```python
from build123d import *

# Parameters (mm, degrees)
SKETCH1_W           = 64
SKETCH1_H           = 54.105
BOSS_EXTRUDE1_DEPTH = 12
SKETCH2_R           = 3.15
CUT_EXTRUDE1_DEPTH  = 85.660209219
FILLET1_R           = 8
SKETCH3_R           = 11
SKETCH3_R_2         = 1.7
CUT_EXTRUDE2_DEPTH  = 85.660209219
CUT_EXTRUDE4_DEPTH  = 8
CUT_EXTRUDE5_START  = -85.903698808
SKETCH6_R           = 3.05
CUT_EXTRUDE5_DEPTH  = 93.903698808


with BuildPart() as part:
    # Sketch1 → Boss-Extrude1 (new body)
    with BuildSketch(Plane.XY):
        with Locations((32, 27.0525)):
            Rectangle(SKETCH1_W, SKETCH1_H)
    extrude(amount=BOSS_EXTRUDE1_DEPTH)

    # Sketch2 → Cut-Extrude1 (cut, through all)
    with BuildSketch(Plane(origin=(0, 0, 0), x_dir=(0, 0, -1), z_dir=(1, 0, 0))):
        with Locations((-6, 46.105)):
            Circle(SKETCH2_R)
        with Locations(Location((-6, 8, 0), (0, 0, 180))):
            Circle(SKETCH2_R)
    extrude(amount=CUT_EXTRUDE1_DEPTH, mode=Mode.SUBTRACT)

    # Fillet1
    fillet1_edges = [part.edges().sort_by_distance(p)[0] for p in [
        (32, 54.105, 0),
        (32, 0, 0),
    ]]
    fillet(fillet1_edges, radius=FILLET1_R)

    # Sketch3 → Cut-Extrude2 (cut, through all)
    with BuildSketch(Plane(origin=(0, 0, 0), x_dir=(-1, 0, 0), z_dir=(0, 0, -1))):
        with Locations((-32, 27.0525)):
            Circle(SKETCH3_R)
        with Locations((-19, 40.0525)):
            Circle(SKETCH3_R_2)
        with Locations((-19, 14.0525)):
            Circle(SKETCH3_R_2)
        with Locations((-45, 14.0525)):
            Circle(SKETCH3_R_2)
        with Locations((-45, 40.0525)):
            Circle(SKETCH3_R_2)
        with BuildLine():
            Line((-8.5, 0), (-8.5, 24.282572203))
            ThreePointArc((-8.5, 24.282572203), (-10.15, 27.0525), (-8.5, 29.822427797))
            Line((-8.5, 29.822427797), (-8.5, 33.0525))
            ThreePointArc((-8.5, 33.0525), (-7, 34.5525), (-5.5, 33.0525))
            Line((-5.5, 33.0525), (-5.5, 29.822427797))
            ThreePointArc((-5.5, 29.822427797), (-3.85, 27.0525), (-5.5, 24.282572203))
            Line((-5.5, 24.282572203), (-5.5, 0))
            Line((-5.5, 0), (-8.5, 0))
        make_face()
    extrude(amount=-CUT_EXTRUDE2_DEPTH, mode=Mode.SUBTRACT)

    # Sketch5 → Cut-Extrude4 (cut)
    with BuildSketch(Plane(origin=(0, 0, 0), x_dir=(-1, 0, 0), z_dir=(0, 0, -1))):
        with BuildLine():
            Line((-19, 17.6525), (-14, 17.6525))
            Line((-14, 17.6525), (-14, 36.4525))
            Line((-14, 36.4525), (-19, 36.4525))
            ThreePointArc((-19, 36.4525), (-21.510876341, 37.472674425), (-22.598679445, 39.955))
            Line((-22.598679445, 39.955), (-22.598679445, 41.7525))
            Line((-22.598679445, 41.7525), (-41.401320555, 41.7525))
            Line((-41.401320555, 41.7525), (-41.401320555, 39.955))
            ThreePointArc((-41.401320555, 39.955), (-42.489123659, 37.472674425), (-45, 36.4525))
            Line((-45, 36.4525), (-50, 36.4525))
            Line((-50, 36.4525), (-50, 17.6525))
            Line((-50, 17.6525), (-45, 17.6525))
            ThreePointArc((-45, 17.6525), (-42.489123659, 16.632325575), (-41.401320555, 14.15))
            Line((-41.401320555, 14.15), (-41.401320555, 12.3525))
            Line((-41.401320555, 12.3525), (-22.598679445, 12.3525))
            Line((-22.598679445, 12.3525), (-22.598679445, 14.15))
            ThreePointArc((-22.598679445, 14.15), (-21.510876341, 16.632325575), (-19, 17.6525))
        make_face()
    extrude(amount=-CUT_EXTRUDE4_DEPTH, mode=Mode.SUBTRACT)

    # Sketch6 → Cut-Extrude5 (cut)
    with BuildSketch(Plane(origin=(0, -0.598076211, 1.035898385), x_dir=(1, 0, 0), z_dir=(0, 0.49999999999999495, -0.8660254037844416)).offset(CUT_EXTRUDE5_START)):
        with Locations(Location((57, -16.92820323, 0), (0, 0, 90))):
            Circle(SKETCH6_R)
    cut_extrude5 = extrude(amount=CUT_EXTRUDE5_DEPTH, mode=Mode.SUBTRACT)

    # Mirror1: Cut-Extrude5 across plane
    add(cut_extrude5.mirror(Plane.ZX.offset(27.0525)), mode=Mode.SUBTRACT)


solid = part.part
```
Part model, mm, in its own coordinate system. A direction names the side the tool comes from. Round coordinates to 2 decimals unless told otherwise and drop trailing zeros. Write each loop counter-clockwise with the first axis right and the second up, starting at its lowest first coordinate (ties: lowest second). Pieces come first, ordered by that corner, then holes. Notation, with made-up numbers: M 56.5,20 L 106.5,20 A13 ccw 106.5,37 Z; hole C 31,-13.75 d9. An arc over 180 degrees is marked long. Answer as CSV lines item,"result". Start each with the question number.
1) Which spindle directions (+Z, -Z, +X, -X, +Y, -Y) get a long thin tool onto all of the face, cutting with end or side? Do faces 5 (the face through (46.7, 14.1, 5.9)), 6 (the face through (56.957, 18.099, 2.593)), 7 (the face through (32, 41.752, 4)). Say none if no direction does.
2) Band-saw the part on C-C (z = 6). Count the separate pieces of the cut face and the enclosed holes in it, then the cut area to 3 significant figures.
3) Mould opens along Y. For faces 1 (the face through (2.71, 5.34, 7.69)), 2 (the face through (5.5, 31, 6)), 3 (the face through (32.45, 51.7, 2.28)), 4 (the face through (3.85, 27.1, 5.92)) say: +Y half, -Y half, draft (parallel to the pull), parting line (faces both ways), or undercut.
4) Drill centre lines: L1, parallel to X at y = 21, z = 0.5; L2, parallel to X at y = 4.5, z = 11; L3, parallel to Z at x = 1.6, y = 8. Where is each one in solid material? Low to high.
5) Band-saw the part on B-B (y = 26). List the corners of the cut face in (x, z).
6) Drop flat-ended pins along their axis: pin 1 (5 mm diameter, centred on y = 45.5, z = 6, fed in from -X); pin 2 (4 mm diameter, centred on x = 40, z = 5, fed in from +Y); pin 3 (4 mm diameter, centred on x = 16, z = 3, fed in from +Y); pin 4 (4 mm diameter, centred on x = 48, z = 3.5, fed in from -Y). Give the stop position or say it passes through.
Worked out:
1,face 5,"+Z, -Z"
1,face 6,"none"
1,face 7,"-Z"
2,separate pieces,"4"
2,enclosed holes,"7"
2,area,"1,540 mm²"
3,face 1,"undercut"
3,face 2,"draft"
3,face 3,"+Y half"
3,face 4,"undercut"
4,L1,"0 to 5.5, 8.5 to 14, 50 to 64"
4,L2,"0 to 5.5, 8.5 to 64"
4,L3,"0 to 2.85, 9.15 to 12"
5,outline,"M 0,0 L 4.03,0 L 4.03,12 L 0,12 Z; M 9.97,0 L 14,0 L 14,8 L 21.05,8 L 21.05,12 L 9.97,12 Z; M 42.95,8 L 50,8 L 50,0 L 64,0 L 64,12 L 42.95,12 Z"
6,pin 1,"through"
6,pin 2,"y = 54.04"
6,pin 3,"y = 53.52"
6,pin 4,"y = 0.4"
